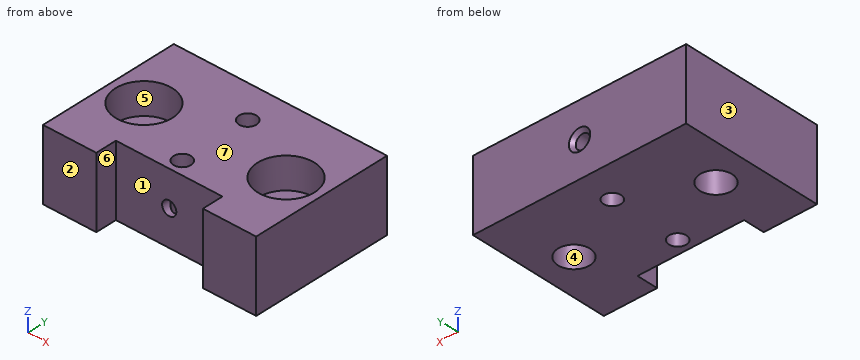
Autodesk Inventor part; units mm, degrees
ref_plane "YZ Plane" through (0, 0, 0) normal (1, 0, 0) x (0, 1, 0)
ref_plane "XZ Plane" through (0, 0, 0) normal (0, 1, 0) x (-1, 0, 0)
ref_plane "XY Plane" through (0, 0, 0) normal (0, 0, 1) x (1, 0, 0)
sketch "Skizze1" plane through (0, 0, 0) normal (0, 0, 1) x (1, 0, 0)
  line L0 (0, 0) -> (30, 0)
  line L1 (30, 0) -> (30, 20)
  line L2 (30, 20) -> (0, 20)
  line L3 (0, 20) -> (0, 0)
  dimension "d0" = 20
  dimension "d1" = 30
extrude "Extrusion1" add sketch "Skizze1" along normal blind 10
sketch "Skizze2" plane through (0, 0, 10) normal (0, 0, 1) x (1, 0, 0)
  line L0 (0, 0) -> (0, 20)
  line L1 (30, 0) -> (0, 0)
  line L2 (30, 20) -> (30, 0)
  line L3 (0, 20) -> (30, 20)
  line L4 (0, 10) -> (30, 10)
  line L5 (15, 20) -> (15, 0)
  point P0 (5, 10)
  point P1 (25, 10)
  dimension "d4" = 20
hole "Bohrung1" at (5, 10, 10) at (25, 10, 10) direction (0, 0, -1) diameter 4.5 end through all counterbore diameter 8 counterbore depth 4.4
sketch "Skizze3" plane through (0, 0, 10) normal (0, 0, 1) x (1, 0, 0)
  circle A0 centre (25, 10) radius 4
  circle A1 centre (5, 10) radius 4
  line L0 (30, 0) -> (0, 0)
  line L1 (0, 20) -> (30, 20)
  line L2 (15, 20) -> (15, 0)
  line L3 (5, 10) -> (25, 10)
  point P0 (15, 15)
  point P1 (15, 5)
  dimension "d12" = 10
hole "Bohrung2" at (15, 15, 10) at (15, 5, 10) direction (0, 0, -1) diameter 2.459 end through all
sketch "Skizze4" plane through (0, 20, 0) normal (0, 1, 0) x (1, 0, 0)
  line L0 (0, -10) -> (30, -10)
  line L1 (30, 0) -> (0, 0)
  line L2 (15, 0) -> (15, -10)
  point P0 (15, -5)
  dimension "d20" = 5
hole "Bohrung3" at (15, 20, 5) direction (0, -1, 0) diameter 2 end through all
chamfer "Fase1" distance 0.5 angle 45 2 edges at (15, 20, 4) (15, 0, 4)
sketch "Skizze5" plane through (0, 0, 0) normal (0, -1, 0) x (1, 0, 0)
  line L0 (30, 10) -> (0, 10)
  line L1 (0, 0) -> (0, 10)
  line L2 (0, 0) -> (30, 0)
  line L3 (7.5, 10) -> (22.5, 10)
  line L4 (22.5, 10) -> (22.5, 0)
  line L5 (22.5, 0) -> (7.5, 0)
  line L6 (7.5, 0) -> (7.5, 10)
  line L7 (15, 10) -> (15, 0)
  dimension "d31" = 15
  dimension "d32" = 15
extrude "Extrusion2" cut sketch "Skizze5" against normal blind 3 contours L4 L2 L7 L0 | L7 L2 L6 L0
properties part number "13_0204_073"
The listing builds one solid part. Answer for the finished solid, in the listing's coordinates (mm). Face numbers are marked on the shaded views. A direction names the side the tool comes from. Coordinates: 2 decimals unless noted, no trailing zeros. Loops run counter-clockwise (first coordinate to the right, second up) from the corner with the lowest first, then second, coordinate; pieces in that order, holes last.
1) A tool of negligible diameter and unlimited length cuts with its end or side. For the marked faces 5, 6 and 7, from which of +Z, -Z, +X, -X, +Y, -Y can it reach the whole face along a straight path? Write none if from no direction.
2) Find section C-C on x = 25. Write down the section's boundary in (y, z).
3) Find section A-A on z = 5. Write down the section's boundary in (x, y).
4) Find section D-D on x = 15. Write down the section's boundary in (y, z), then the cut area to 3 significant figures.
5) Find the intervals of material crossed by L1, parallel to X at y = 10, z = 2.7; L2, parallel to X at y = 1, z = 2.5; L3, parallel to X at y = 3.3, z = 5, in increasing order.
6) Determine the mould class of the marked faces 1, 2, 3 and 4 for opening direction X: pulls with the +X half, pulls with the -X half, needs draft (parallel to the pull), parting line crosses it, or undercut.
7) Find section B-B on y = 10. Write down the section's boundary in (x, z), then the cut area to 3 significant figures.
8) Flat-ended cylindrical pins translate along their axes: pin 1 Ø10.5 at (x, y) = (25, 10) entering from +Z; pin 2 Ø2.5 at (x, z) = (15, 5) entering from +Y. Find the tip coordinate at first contact, or state that the pin passes through.
Values:
1. face 5: +Z
1. face 6: +Z, -Z, -Y
1. face 7: +Z, +X, -X, +Y, -Y
2. outline: (0, 0) - (7.75, 0) - (7.75, 5.6) - (6, 5.6) - (6, 10) - (0, 10) - close; (12.25, 0) - (20, 0) - (20, 10) - (14, 10) - (14, 5.6) - (12.25, 5.6) - close
3. outline: (0, 0) - (7.5, 0) - (7.5, 3) - (14, 3) - (14, 4.28) arc R1.23 cw to (14, 5.72) - (14, 14.28) arc R1.23 cw to (14, 15.72) - (14, 19.5) - (13.5, 20) - (0, 20) - close; (16, 3) - (22.5, 3) - (22.5, 0) - (30, 0) - (30, 20) - (16.5, 20) - (16, 19.5) - (16, 15.72) arc R1.23 cw to (16, 14.28) - (16, 5.72) arc R1.23 cw to (16, 4.28) - close; hole circle Ø4.5 at (5, 10); hole circle Ø4.5 at (25, 10)
4. outline: (3, 0) - (3.77, 0) - (3.77, 4) - (3, 4) - close; (3, 6) - (3.77, 6) - (3.77, 10) - (3, 10) - close; (6.23, 0) - (13.77, 0) - (13.77, 4) - (6.23, 4) - close; (6.23, 6) - (13.77, 6) - (13.77, 10) - (6.23, 10) - close; (16.23, 0) - (20, 0) - (20, 3.5) - (19.5, 4) - (16.23, 4) - close; (16.23, 6) - (19.5, 6) - (20, 6.5) - (20, 10) - (16.23, 10) - close
4. area: 96.4 mm2
5. L1: x = 0 to 2.75, 7.25 to 22.75, 27.25 to 30
5. L2: x = 0 to 7.5, 22.5 to 30
5. L3: x = 0 to 14, 16 to 30
6. face 1: undercut
6. face 2: needs draft
6. face 3: pulls with the -X half
6. face 4: undercut
7. outline: (0, 0) - (2.75, 0) - (2.75, 5.6) - (1, 5.6) - (1, 10) - (0, 10) - close; (7.25, 0) - (22.75, 0) - (22.75, 5.6) - (21, 5.6) - (21, 10) - (9, 10) - (9, 5.6) - (7.25, 5.6) - close; (27.25, 0) - (30, 0) - (30, 10) - (29, 10) - (29, 5.6) - (27.25, 5.6) - close; hole circle Ø2 at (15, 5)
7. area: 176 mm2
8. pin 1: stops at z = 10
8. pin 2: stops at y = 19.75
